```python
from build123d import *

# Parameters (mm, degrees)
SKETCH001_W  = 1
SKETCH001_H  = 8.5
POCKET_DEPTH = 1.2


with BuildPart() as part:
    # Sketch → Revolution (revolve)
    with BuildSketch(Plane.YZ):
        Polygon((0, 0), (0, 3.75), (0.5, 4.25), (2.4, 4.25), (2.4, 2.75), (12.4, 2.75), (12.4, 1.57), (14.601739, 1.57), (14.85, 2), (18.151739, 2), (18.4, 1.57), (18.4, 0), align=None)
    revolve(axis=Axis((0, 0, 0), (0, 1, 0)))

    # Sketch001 → Pocket (cut)
    with BuildSketch(Plane(origin=(0, 0, 0), x_dir=(0, 0, -1), z_dir=(0, -1, 0))):
        Rectangle(SKETCH001_W, SKETCH001_H)
    extrude(amount=-POCKET_DEPTH, mode=Mode.SUBTRACT)


solid = part.part
```
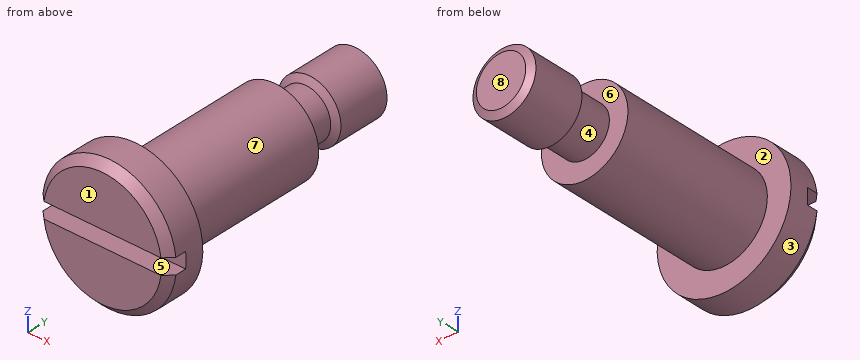
Part model, mm, in its own coordinate system. Face numbers are marked on the shaded views. A direction names the side the tool comes from. Give positions to 0.01 mm unless a question says otherwise; leave off trailing zeros. Loops run counter-clockwise (first coordinate to the right, second up) from the corner with the lowest first, then second, coordinate; pieces in that order, holes last. Notation, with made-up numbers: M -26,38 L -9,38 A25 cw -9,76 Z; hole C -40,37.5 d2. An arc over 180 degrees is marked long. Return JSON: item names as keys, results as strings.
1) Saw through at C-C, the plane y = 17. List the corners of the cut face in (x, z).
Calculated:
{"outline": "C 0,0 d4"}
2) 3-axis set-ups, long thin cutter, end or side, ignore diameter. For the marked faces 1, 2, 3, 4 and 5: which of +Z, -Z, +X, -X, +Y, -Y reach the whole face in a straight line?
Calculated:
{"face 1": "+Z, -Z, +X, -X, -Y", "face 2": "+Y", "face 3": "+Y, -Y", "face 4": "none", "face 5": "+X, -X, -Y"}
3) Pull direction Y, two halves, no side cores. Call the marked faces 6, 7 and 8: released by +Y, released by -Y, zero draft, split by the parting line, or undercut.
Calculated:
{"face 6": "undercut", "face 7": "zero draft", "face 8": "released by +Y"}
4) Flat gauge pins, fed straight in: pin 1 Ø1 at (y, z) = (4, 1.5) entering from -X; pin 2 Ø2 at (x, y) = (0, 10) entering from +Z; pin 3 Ø1 at (x, y) = (-1, 0.5) entering from +Z. Where does each tip first touch, or does it go through?
Calculated:
{"pin 1": "stops at x = -2.56", "pin 2": "stops at z = 2.75", "pin 3": "stops at z = 4.22"}
5) Saw through at D-D, the plane y = 8. List the corners of the cut face in (x, z).
Calculated:
{"outline": "C 0,0 d5.5"}
6) Saw through at B-B, the plane x = 0. List the corners of the cut face in (y, z).
Calculated:
{"outline": "M 0,-3.75 L 0.5,-4.25 L 2.4,-4.25 L 2.4,-2.75 L 12.4,-2.75 L 12.4,-1.57 L 14.6,-1.57 L 14.85,-2 L 18.15,-2 L 18.4,-1.57 L 18.4,1.57 L 18.15,2 L 14.85,2 L 14.6,1.57 L 12.4,1.57 L 12.4,2.75 L 2.4,2.75 L 2.4,4.25 L 0.5,4.25 L 0,3.75 L 0,0.5 L 1.2,0.5 L 1.2,-0.5 L 0,-0.5 Z"}
7) Saw through at A-A, the plane z = 0. List the corners of the cut face in (x, y), then the cut area to 3 significant figures.
Calculated:
{"outline": "M -4.25,1.2 L 4.25,1.2 L 4.25,2.4 L 2.75,2.4 L 2.75,12.4 L 1.57,12.4 L 1.57,14.6 L 2,14.85 L 2,18.15 L 1.57,18.4 L -1.57,18.4 L -2,18.15 L -2,14.85 L -1.57,14.6 L -1.57,12.4 L -2.75,12.4 L -2.75,2.4 L -4.25,2.4 Z", "area": "87.1 mm2"}
8) Drill centre lines: line 1 (Y direction, x = -3, z = -0.75); line 2 (Y direction, x = -0.25, z = 2.5); line 3 (Z direction, x = -2.5, y = 3). Where is each one in solid material? Low to high.
Calculated:
{"line 1": "y = 0 to 2.4", "line 2": "y = 0 to 12.4", "line 3": "z = -1.15 to 1.15"}
